The figure shows three views and two pictorial views of one solid part (mm, origin at its lowest corner). Answer the questions. A direction names the side the tool comes from. Round coordinates to 2 decimals unless told otherwise and drop trailing zeros. Loops run counter-clockwise (first coordinate to the right, second up) from the corner with the lowest first, then second, coordinate; pieces in that order, holes last. Notation, with made-up numbers: (71, 18) -> (82, 18) arc R33 cw to (82, 55) -> close; hole circle Ø9 at (77.25, 11). An arc over 180 degrees is marked (long way). Use a Markdown table: item, result. Add a question column.
Q1. Which of the six approach directions +Z, -Z, +X, -X, +Y, -Y give full straight-line access (tool end or side, diameter ignored) to the marked faces 1, 2 and 3?
Q2. For a pull along X with two mould halves and no side action, classify the marked faces 4, 5 and 6 as released by +X, released by -X, zero draft, split by the parting line, or undercut.
Q3. Consider line 1 (Z direction, x = 22.75, y = 9); line 2 (X direction, y = 9, z = 11.5); line 3 (Y direction, x = 14, z = 39.3). Determine where each line is inside the solid, lowest interval first.
Q4. Given pin 1 Ø11.5 at (x, y) = (15.5, 15.5) entering from -Z; pin 2 Ø1 at (x, y) = (7.5, 17.5) entering from +Z; pin 3 Ø5 at (x, y) = (24.5, 9) entering from -Z, each flat-ended and moving along its own axis, determine where each tip first touches the part or whether it passes through.
Q5. Section C-C on x = 14 is taken. Give the vertices of the cut face in (y, z) (3 decimals), then the cut area to 3 significant figures.
Q6. Section D-D on x = 20.25 is taken. Give the vertices of the cut face in (y, z), then the cut area to 3 significant figures.
Q7. Section A-A on y = 12 is taken. Give the vertices of the cut face in (x, z) (3 decimals), then the cut area to 3 significant figures.
Q8. Section B-B on z = 30.5 is taken. Give the vertices of the cut face in (x, y).
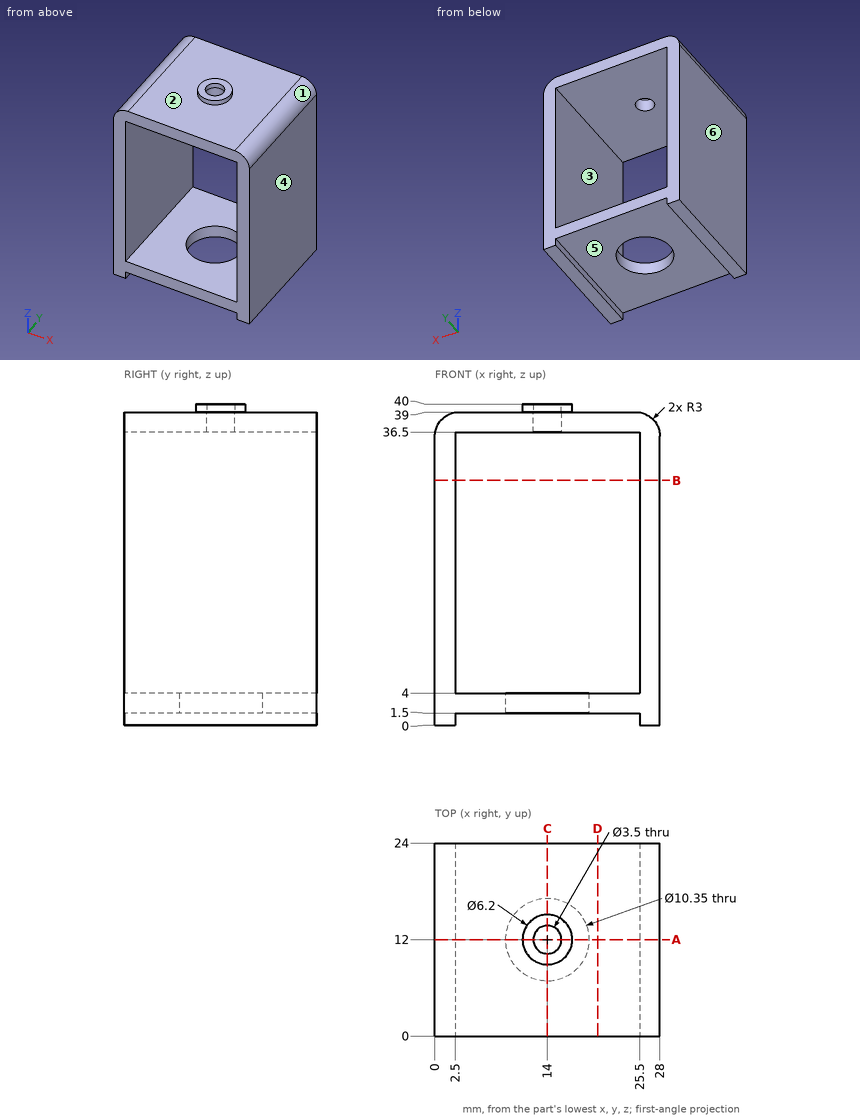
Checked values:
| question | item | result |
|---|---|---|
| 1 | face 1 | +Z, +X, +Y, -Y |
| 1 | face 2 | +Z |
| 1 | face 3 | +Y, -Y |
| 2 | face 4 | released by +X |
| 2 | face 5 | undercut |
| 2 | face 6 | released by -X |
| 3 | line 1 | z = 1.5 to 4, 36.5 to 39 |
| 3 | line 2 | x = 0 to 2.5, 25.5 to 28 |
| 3 | line 3 | y = 8.9 to 10.25, 13.75 to 15.1 |
| 4 | pin 1 | stops at z = 1.5 |
| 4 | pin 2 | stops at z = 39 |
| 4 | pin 3 | stops at z = 0 |
| 5 | outline | (0, 1.5) -> (6.825, 1.5) -> (6.825, 4) -> (0, 4) -> close; (0, 36.5) -> (10.25, 36.5) -> (10.25, 40) -> (8.9, 40) -> (8.9, 39) -> (0, 39) -> close; (13.75, 36.5) -> (24, 36.5) -> (24, 39) -> (15.1, 39) -> (15.1, 40) -> (13.75, 40) -> close; (17.175, 1.5) -> (24, 1.5) -> (24, 4) -> (17.175, 4) -> close |
| 5 | area | 88.1 mm2 |
| 6 | outline | (0, 1.5) -> (24, 1.5) -> (24, 4) -> (0, 4) -> close; (0, 36.5) -> (24, 36.5) -> (24, 39) -> (0, 39) -> close |
| 6 | area | 120 mm2 |
| 7 | outline | (0, 0) -> (2.5, 0) -> (2.5, 1.5) -> (8.825, 1.5) -> (8.825, 4) -> (2.5, 4) -> (2.5, 36.5) -> (12.25, 36.5) -> (12.25, 40) -> (10.9, 40) -> (10.9, 39) -> (3, 39) arc R3 ccw to (0, 36) -> close; (15.75, 36.5) -> (25.5, 36.5) -> (25.5, 4) -> (19.175, 4) -> (19.175, 1.5) -> (25.5, 1.5) -> (25.5, 0) -> (28, 0) -> (28, 36) arc R3 ccw to (25, 39) -> (17.1, 39) -> (17.1, 40) -> (15.75, 40) -> close |
| 7 | area | 274 mm2 |
| 8 | outline | (0, 0) -> (2.5, 0) -> (2.5, 24) -> (0, 24) -> close; (25.5, 0) -> (28, 0) -> (28, 24) -> (25.5, 24) -> close |
